```python
from build123d import *

# Parameters (mm, degrees)
F1_DEPTH       = 25
F0_R           = 7.5
F2_DEPTH       = 3
F3_D           = 6.5
F3_DEPTH       = 3.001
F4_D           = 4.5
F4_DEPTH       = 25
F4_CBORE_D     = 6.5
F4_CBORE_DEPTH = 23
F4_TIP         = 1.3519363928
F5_SIZE        = 0.99999


# Not quite as in the source:
# - a fillet or chamfer is up to 0.001 mm smaller than in the source, because OpenCascade refuses the exact size


with BuildPart() as f1:
    # F0 (on Top) → F1 (new body)
    with BuildSketch(Plane.XY):
        with BuildLine():
            Line((-3.5, 2.8284271247), (-3.5, -2.8284271247))
            ThreePointArc((-3.5, -2.8284271247), (4.5, 0), (-3.5, 2.8284271247))
        make_face()
    extrude(amount=F1_DEPTH)

    # F0 (on Top) → F2 (join)
    with BuildSketch(Plane.XY):
        Circle(F0_R)
        with BuildLine():
            ThreePointArc((-3.5, 2.8284271247), (4.5, 0), (-3.5, -2.8284271247))
            Line((-3.5, -2.8284271247), (-3.5, 2.8284271247))
        make_face(mode=Mode.SUBTRACT)
        with BuildLine():
            Line((-3.5, 2.8284271247), (-3.5, -2.8284271247))
            ThreePointArc((-3.5, -2.8284271247), (4.5, 0), (-3.5, 2.8284271247))
        make_face()
    extrude(amount=-F2_DEPTH)

    # F3 (through all, one way)
    with BuildSketch(Plane.XY):
        with Locations((0, 0)):
            Circle(F3_D / 2)
    extrude(amount=-F3_DEPTH, mode=Mode.SUBTRACT)

    # F4
    with Locations(Plane(origin=(0, 0, 0), x_dir=(1, 0, 0), z_dir=(0, 0, -1))):
        with Locations((0, 0)):
            CounterBoreHole(F4_D / 2, F4_CBORE_D / 2, F4_CBORE_DEPTH, depth=F4_DEPTH)
            with Locations((0, 0, -(F4_DEPTH + F4_TIP / 2))):  # 118° drill point
                Cone(0, F4_D / 2, F4_TIP, mode=Mode.SUBTRACT)

    # F5 (size 1 in the source; OpenCascade refuses exactly that, so slightly less here)
    f5_edges = [f1.edges().sort_by_distance(p)[0] for p in [
        (4.5, 0, 25),
        (-2.25, 0, 23),
    ]]
    chamfer(f5_edges, length=F5_SIZE)


solid = f1.part
```
Work out the finished part from the listing and answer in its coordinate system (mm). A direction names the side the tool comes from. Give positions to 0.01 mm unless a question says otherwise; leave off trailing zeros. Loops run counter-clockwise (first coordinate to the right, second up) from the corner with the lowest first, then second, coordinate; pieces in that order, holes last. Notation, with made-up numbers: (41.5, 63.5) -> (88.5, 63.5) arc R9 cw to (88.5, 74.5) -> close; hole circle Ø8 at (84.5, 38.25). An arc over 180 degrees is marked (long way). Put each result on its own line as item: value. Start each with the question number.
Item 1: Find the intervals of material crossed by L1, parallel to X at y = 0, z = 16.5; L2, parallel to Y at x = 0, z = 3; L3, parallel to X at y = 0, z = 24.35, in increasing order. Write a range as [from, to].
Item 2: The part is cut by section B-B (z = 8.5). Give the vertices of the cut face in (x, y), then the cut area to 3 significant figures.
Item 3: Each of these flat-tipped pins is pushed along its axis until it touches: P1, Ø1, axis at x = 1.5, y = -1, coming from the +Z side; P2, Ø5, axis at x = -4.5, z = 19.5, coming from the +Y side; P3, Ø4, axis at x = 0, y = 0, coming from the -Z side; P4, Ø1.7, axis at y = 0, z = 18, coming from the -X side. Where does it stop, or does it pass through?
Item 4: The part is cut by section C-C (x = 5). Give the vertices of the cut face in (y, z), then the cut area to 3 significant figures.
Item 5: The mould has two halves that part along Y. Classify faces 1 (the face through (2.3, -0.7, 25)), 2 (the face through (3.67, -0.161, 24.826)), 3 (the face through (0.29, -2.23, 24.51)), 4 (the face through (-2.579, -1.978, 10.182)): released by +Y, released by -Y, zero draft, split by the parting line, or undercut.
Item 6: Which of the six approach directions +Z, -Z, +X, -X, +Y, -Y give full straight-line access (tool end or side, diameter ignored) to faces 5 (the face through (-3.5, 0, 12)), 6 (the face through (0, -5, 0)), 7 (the face through (2, -3, -3))?
Answers below:
1. L1: [-3.5, -3.25], [3.25, 4.5]
1. L2: [-4.5, -3.25], [3.25, 4.5]
1. L3: [-3.5, -2.25], [2.25, 4.15]
2. outline: (-3.5, -2.83) arc R4.5 ccw (long way) to (-3.5, 2.83) -> close; hole circle Ø6.5 at (0, 0)
2. area: 26.6 mm2
3. P1: z = 25
3. P2: y = 4.03
3. P3: through
3. P4: x = -3.5
4. outline: (-5.59, -3) -> (5.59, -3) -> (5.59, 0) -> (-5.59, 0) -> close
4. area: 33.5 mm2
5. face 1: zero draft
5. face 2: split by the parting line
5. face 3: undercut
5. face 4: undercut
6. face 5: +Z, -X, +Y, -Y
6. face 6: +Z
6. face 7: -Z, +X, -X, +Y, -Y
